Build history of the part. All positions in model axes, mm. A direction names the side the tool comes from. Give positions to 0.01 mm unless a question says otherwise; leave off trailing zeros. Write each loop counter-clockwise with the first axis right and the second up, starting at its lowest first coordinate (ties: lowest second). Pieces come first, ordered by that corner, then holes.
Autodesk Inventor part; units mm, degrees
ref_plane "YZ Plane" through (0, 0, 0) normal (1, 0, 0) x (0, 1, 0)
ref_plane "XZ Plane" through (0, 0, 0) normal (0, 1, 0) x (-1, 0, 0)
ref_plane "XY Plane" through (0, 0, 0) normal (0, 0, 1) x (1, 0, 0)
sketch "Sketch1" plane through (0, 0, 0) normal (0, 1, 0) x (-1, 0, 0)
  line L0 (0, 0) -> (-100, 0)
  line L1 (-100, 0) -> (-100, -100)
  line L2 (-100, -100) -> (0, -100)
  line L3 (0, -100) -> (0, 0)
  dimension "d0" = 100
  dimension "d1" = 100
extrude "base" add sketch "Sketch1" along normal blind 9
sketch "Sketch2" plane through (0, 9, 0) normal (0, 1, 0) x (1, 0, 0)
  circle A0 centre (96, 25) radius 1.75
  line L0 (100, 0) -> (100, 100)
  circle A1 centre (69, 25) radius 1.75
  line L1 (0, 0) -> (100, 0)
  line L2 (100, 50) -> (95, 50)
  circle A2 centre (96, 75) radius 1.75
  circle A3 centre (69, 75) radius 1.75
  line L3 (63, 0) -> (63, 100)
  line L4 (100, 100) -> (0, 100)
  line L5 (100, 25) -> (100, 11)
  line L6 (100, 11) -> (63, 11)
  line L7 (100, 89) -> (63, 89)
  circle A4 centre (82, 25) radius 17.5
  point P0 (63, 89)
  dimension "d6" = 4
  dimension "d7" = 3.5
  dimension "d9" = 3.5
  dimension "d10" = 27
  dimension "d11" = 25
  dimension "d13" = 37
  dimension "d14" = 14
  dimension "d17" = 35
extrude "wheel space" cut sketch "Sketch2" against normal through all contours A0 | L1 L3 L6 A4 L0 | A4 L6 | L3 L4 L0 L7 | A1 | A2 | A3 picked at (84.4264, 10.3619)
sketch "Sketch3" plane through (0, 0, 0) normal (0, 0, 1) x (1, 0, 0)
  line L0 (63, 9) -> (0, 9)
  line L1 (0, 0) -> (0, 9)
  line L2 (63, 0) -> (0, 0)
  line L3 (5, 9) -> (0, 0)
  dimension "d18" = 5
extrude "ramp" cut sketch "Sketch3" against normal through all
sketch "Sketch4" plane through (0, 9, 0) normal (0, 1, 0) x (1, 0, 0)
  circle A0 centre (69, 75) radius 1.75
  circle A1 centre (96, 25) radius 1.75
  circle A2 centre (96, 75) radius 1.75
  circle A3 centre (69, 25) radius 1.75
  line L0 (5, 100) -> (5, 0)
  line L1 (5, 0) -> (63, 0)
  line L2 (63, 0) -> (63, 11)
  line L3 (63, 11) -> (100, 11)
  line L4 (100, 11) -> (100, 89)
  line L5 (100, 89) -> (63, 89)
  line L6 (63, 89) -> (63, 100)
  line L7 (63, 100) -> (5, 100)
  line L8 (63, 100) -> (63, 89)
  line L9 (61, 95) -> (10, 95)
  line L10 (10, 95) -> (10, 5)
  line L11 (10, 5) -> (63, 5)
  line L12 (63, 11) -> (63, 0)
  line L13 (63, 89) -> (61, 89)
  line L14 (61, 89) -> (61, 95)
  line L15 (63, 5) -> (53, 5)
  line L16 (53, 5) -> (53, 7)
  line L17 (53, 7) -> (63, 7)
  line L18 (63, 7) -> (63, 5)
  point P0 (0, 0)
  point P1 (63, 95)
  dimension "d21" = 5
  dimension "d22" = 5
  dimension "d23" = 5
  dimension "d64" = 2
  dimension "d72" = 10
  dimension "d73" = 2
extrude "walls" add sketch "Sketch4" along normal blind 5 contours L7 L6 L13 L14 L9 L10 L11 L2 L1 L0 | L11 L16 L17 L2
sketch "Sketch5" plane through (0, 9, 0) normal (0, 1, 0) x (1, 0, 0)
  line L0 (22.7322, 84.5) -> (12.7322, 84.5)
  line L1 (12.7322, 84.5) -> (12.7322, 44.5)
  line L2 (12.7322, 44.5) -> (22.7322, 44.5)
  line L3 (22.7322, 44.5) -> (22.7322, 84.5)
  line L4 (14.7322, 44.5) -> (20.7322, 44.5)
  line L5 (20.7322, 44.5) -> (20.7322, 55.5)
  line L6 (20.7322, 55.5) -> (14.7322, 55.5)
  line L7 (14.7322, 55.5) -> (14.7322, 44.5)
  line L8 (14.7322, 44.5) -> (20.7322, 55.5) construction
  line L9 (20.7322, 44.5) -> (14.7322, 55.5) construction
  line L10 (10, 5) -> (10, 95)
  circle A0 centre (17.7322, 64) radius 1.75
  line L11 (100, 84.5) -> (90, 84.5)
  line L12 (90, 84.5) -> (90, 44.5)
  line L13 (90, 44.5) -> (100, 44.5)
  line L14 (100, 44.5) -> (100, 84.5)
  line L15 (92, 44.5) -> (98, 44.5)
  line L16 (98, 44.5) -> (98, 55.5)
  line L17 (98, 55.5) -> (92, 55.5)
  line L18 (92, 55.5) -> (92, 44.5)
  line L19 (92, 44.5) -> (98, 55.5) construction
  line L20 (98, 44.5) -> (92, 55.5) construction
  circle A1 centre (95, 64) radius 1.75
  circle A2 centre (96, 75) radius 1.75
  line L21 (100, 11) -> (100, 89)
  circle A3 centre (95, 36) radius 1.75
  circle A4 centre (17.7322, 36) radius 1.75
  line L22 (100, 57.5) -> (90, 57.5)
  line L23 (90, 57.5) -> (90, 42.5)
  line L24 (90, 42.5) -> (100, 42.5)
  line L25 (100, 42.5) -> (100, 57.5)
  line L26 (100, 57.5) -> (90, 42.5) construction
  line L27 (90, 57.5) -> (100, 42.5) construction
  point P0 (0, 0)
  point P1 (17.7322, 50)
  point P2 (10, 50)
  point P3 (17.7322, 50)
  point P4 (95, 50)
  point P5 (95, 50)
  point P6 (95, 50)
  point P7 (17.7322, 50)
  point P8 (92, 44.5)
  point P9 (98, 44.5)
  point P10 (95, 84.5)
  dimension "d26" = 10
  dimension "d27" = 40
  dimension "d28" = 5.5
  dimension "d29" = 6
  dimension "d30" = 11
  dimension "d31" = 3.5
  dimension "d32" = 14
  dimension "d33" = 10
  dimension "d34" = 40
  dimension "d35" = 5.5
  dimension "d36" = 6
  dimension "d37" = 11
  dimension "d38" = 3.5
  dimension "d39" = 14
  dimension "d60" = 3.5
  dimension "d61" = 14
  dimension "d62" = 3.5
  dimension "d63" = 14
  dimension "d65" = 10
  dimension "d66" = 15
extrude "ir sensor" cut sketch "Sketch5" against normal through all contours L2 L7 L6 L5 | A0 | L13 L18 L17 L16 | A1 | A3 | A4
sketch "Sketch8" plane through (0, 14, 0) normal (0, 1, 0) x (1, 0, 0)
  line L0 (61, 89) -> (63, 89)
  line L1 (63, 89) -> (63, 100)
  line L2 (63, 100) -> (5, 100)
  line L3 (5, 100) -> (5, 0)
  line L4 (5, 0) -> (63, 0)
  line L5 (63, 0) -> (63, 7)
  line L6 (63, 7) -> (53, 7)
  line L7 (53, 7) -> (53, 5)
  line L8 (53, 5) -> (10, 5)
  line L9 (10, 5) -> (10, 95)
  line L10 (10, 95) -> (61, 95)
  line L11 (61, 95) -> (61, 89)
  circle A0 centre (7.5, 85) radius 1.25
  circle A1 centre (7.5, 15) radius 1.25
  circle A2 centre (48, 2.5) radius 1.25
  circle A3 centre (48, 97.5) radius 1.25
  point P0 (0, 0)
  dimension "d82" = 2.5
  dimension "d84" = 2.5
  dimension "d85" = 2.5
  dimension "d87" = 2.5
  dimension "d88" = 15
  dimension "d89" = 15
  dimension "d90" = 15
  dimension "d91" = 2.5
  dimension "d92" = 2.5
  dimension "d93" = 2.5
sketch "Sketch6" plane through (0, 9, 0) normal (0, 1, 0) x (1, 0, 0)
  line L0 (20.7322, 44.5) -> (14.7322, 44.5)
  circle A0 centre (17.7322, 64) radius 1.75
  line L1 (53, 5) -> (10, 5)
  line L2 (10, 95) -> (61, 95)
  circle A1 centre (69, 25) radius 1.75
  circle A2 centre (96, 25) radius 1.75
  circle A3 centre (69, 25) radius 1.75
  circle A4 centre (96, 25) radius 1.75
  line L3 (69, 25) -> (96, 25)
  circle A5 centre (30, 25) radius 1.25
  line L4 (10, 5) -> (10, 95)
  circle A6 centre (30, 59.5) radius 1.25
  circle A7 centre (48, 97.5) radius 1.25
  circle A8 centre (48, 2.5) radius 1.25
  circle A9 centre (7.5, 85) radius 1.25
  circle A10 centre (7.5, 15) radius 1.25
  point P0 (0, 0)
  point P1 (63, 5)
  point P2 (63, 95)
  dimension "d75" = 2.5
  dimension "d76" = 20
  dimension "d77" = 20
  dimension "d79" = 2.5
  dimension "d80" = 34.5
extrude "mount holes" cut sketch "Sketch6" against normal through all both and the other way through all contours A5 | A6 | A7 | A8 | A9 | A10
sketch "Sketch7" plane through (0, 0, 0) normal (0, -1, 0) x (1, 0, 0)
  line L0 (92, -44.5) -> (98, -44.5)
  line L1 (98, -44.5) -> (98, -55.5)
  line L2 (98, -55.5) -> (92, -55.5)
  line L3 (92, -55.5) -> (92, -44.5)
  circle A0 centre (17.7322, -64) radius 1.75
  circle A1 centre (95, -64) radius 1.75
  line L4 (20.7322, -44.5) -> (20.7322, -55.5)
  line L5 (20.7322, -55.5) -> (14.7322, -55.5)
  line L6 (14.7322, -55.5) -> (14.7322, -44.5)
  line L7 (14.7322, -44.5) -> (20.7322, -44.5)
  circle A2 centre (69, -75) radius 1.75
  circle A3 centre (96, -25) radius 1.75
  circle A4 centre (96, -75) radius 1.75
  circle A5 centre (69, -25) radius 1.75
  line L8 (63, -100) -> (63, -89)
  line L9 (63, -89) -> (100, -89)
  line L10 (100, -11) -> (100, -89)
  line L11 (100, -11) -> (63, -11)
  line L12 (63, -11) -> (63, 0)
  line L13 (0, 0) -> (63, 0)
  line L14 (0, -100) -> (0, 0)
  line L15 (63, -100) -> (0, -100)
  circle A6 centre (69, -75) radius 6
  circle A7 centre (69, -25) radius 1.75
  circle A8 centre (69, -25) radius 6
  circle A9 centre (96, -25) radius 1.75
  circle A10 centre (17.7322, -64) radius 6
  circle A11 centre (95, -36) radius 1.75
  arc A12 (89, -36) -> (95, -42) centre (95, -36) ccw
  line L16 (98, -31) -> (98.3166, -31)
  line L17 (100, -11) -> (100, -89)
  line L18 (96, -19) -> (100, -19)
  line L19 (100, -50) -> (98.3161, -50)
  line L20 (95, -42) -> (100, -42)
  circle A13 centre (17.7322, -36) radius 1.75
  circle A14 centre (17.7322, -36) radius 6
  line L21 (92, -19) -> (96, -19)
  line L22 (89, -36) -> (89, -19)
  line L23 (89, -19) -> (92, -19)
  circle A15 centre (96, -75) radius 1.75
  circle A16 centre (96, -75) radius 1.75
  circle A17 centre (95, -64) radius 1.75
  arc A18 (95, -58) -> (89, -64) centre (95, -64) ccw
  line L24 (98, -69) -> (98.3166, -69)
  line L25 (96, -81) -> (100, -81)
  line L26 (95, -58) -> (100, -58)
  line L27 (92, -81) -> (96, -81)
  line L28 (89, -64) -> (89, -81)
  line L29 (89, -81) -> (92, -81)
  circle A19 centre (30, -59.5) radius 1.25
  circle A20 centre (30, -25) radius 1.25
  circle A21 centre (30, -59.5) radius 6
  circle A22 centre (30, -25) radius 6
  circle A23 centre (48, -97.5) radius 1.25
  circle A24 centre (48, -2.5) radius 1.25
  circle A25 centre (7.5, -15) radius 1.25
  circle A26 centre (7.5, -85) radius 1.25
  arc A27 (52, -97.5) -> (44, -97.5) centre (48, -97.5) ccw
  line L30 (44, -97.5) -> (44, -100)
  line L31 (63, -100) -> (5, -100)
  line L32 (52, -97.5) -> (52, -100)
  line L33 (44, -2.5) -> (44, 0)
  line L34 (0, 0) -> (63, 0)
  line L35 (52, -2.5) -> (52, 0)
  circle A28 centre (7.5, -15) radius 4
  circle A29 centre (7.5, -85) radius 4
  arc A30 (44, -2.5) -> (52, -2.5) centre (48, -2.5) ccw
  point P0 (100, -31)
  point P1 (96, -31)
  point P2 (93.1644, -30.2877)
  point P3 (96, -69)
  point P4 (93.1644, -69.7123)
  dimension "d69" = 12
  dimension "d71" = 12
  dimension "d94" = 8
  dimension "d96" = 8
  dimension "d97" = 8
extrude "mount holes flush" cut sketch "Sketch7" against normal blind 4 contours L15 L30 A27 L32 | L25 L27 L29 L28 A18 L26 L10 | L20 A12 L22 L23 L21 L18 L10 | L13 L35 A30 L33 | A6 | A8 | A10 | A14 | A20 | A21 | A22 | A28 | A29
extrude "Extrusion8" add sketch "Sketch5" along normal blind 3 contours L14 L13 L16 L17 L18 L12 L22 | L21 L24 L23 L13
properties part number "jeff"
1. Saw through at B-B on z = -75. Give the cut face in (x, y).
2. 3-axis set-ups, long thin cutter, end or side, ignore diameter. For faces 5 (the face through (95, 6, -55.5)), 6 (the face through (94, 4, -30)), 7 (the face through (8, 14, -47)), 8 (the face through (48.1, 2, -93.5)), 9 (the face through (7, 4, -17)): which of +Z, -Z, +X, -X, +Y, -Y reach the whole face in a straight line?
3. Drill centre lines: line 1 along Z through (x, y) = (69, 6.75); line 2 along Z through (x, y) = (48, 13); line 3 along Z through (x, y) = (56, 12). Where is each one in solid material? Low to high.
4. Mould opens along X. For faces 1 (the face through (90.804, 1.972, -59.711)), 2 (the face through (94, 2, -19)), 3 (the face through (47.84, 9.07, -98.74)), 4 (the face through (5, 11, -51)) say: pulls with the +X half, pulls with the -X half, needs draft (parallel to the pull), parting line crosses it, or undercut.
5. Saw through at C-C on x = 68.5. Give the cut face in (y, z), plus the area to 3 significant figures.
6. Saw through at A-A on y = 10.5. Give the cut face in (x, z).
7. Saw through at D-D on z = -39.5. Give the cut face in (x, y).
8. Drop flat-ended pins along their axis: pin 1 (4.5 mm diameter, centred on x = 82.5, y = 5.5, fed in from +Z); pin 2 (7 mm diameter, centred on x = 30, z = -59.5, fed in from +Y); pin 3 (6 mm diameter, centred on x = 16, z = -38, fed in from -Y). Give the stop position or say it passes through.
Outcome:
1. outline: (0, 0) - (63, 0) - (63, 4) - (67.25, 4) - (67.25, 9) - (10, 9) - (10, 14) - (5, 14) - (5, 9) - close; (70.75, 4) - (75, 4) - (75, 0) - (89, 0) - (89, 4) - (94.25, 4) - (94.25, 9) - (70.75, 9) - close; (97.75, 4) - (100, 4) - (100, 9) - (97.75, 9) - close
2. face 5: +Y, -Y
2. face 6: +X, -Y
2. face 7: +Z, -Z, +X, -X, +Y
2. face 8: -Z, -Y
2. face 9: -Y
3. line 1: z = -89 to -76.75, -73.25 to -26.75, -23.25 to -11
3. line 2: z = -100 to -98.75, -96.25 to -95, -5 to -3.75, -1.25 to 0
3. line 3: z = -100 to -95, -7 to 0
4. face 1: pulls with the +X half
4. face 2: needs draft
4. face 3: undercut
4. face 4: pulls with the -X half
5. outline: (0, -89) - (9, -89) - (9, -76.68) - (4, -76.68) - (4, -80.98) - (0, -80.98) - close; (0, -69.02) - (4, -69.02) - (4, -73.32) - (9, -73.32) - (9, -26.68) - (4, -26.68) - (4, -30.98) - (0, -30.98) - close; (0, -19.02) - (4, -19.02) - (4, -23.32) - (9, -23.32) - (9, -11) - (0, -11) - close
5. area: 573 mm2
6. outline: (5, -100) - (63, -100) - (63, -89) - (61, -89) - (61, -95) - (10, -95) - (10, -5) - (53, -5) - (53, -7) - (63, -7) - (63, 0) - (5, 0) - close; (90, -57.5) - (100, -57.5) - (100, -42.5) - (90, -42.5) - close; hole circle Ø2.5 at (7.5, -85); hole circle Ø2.5 at (7.5, -15); hole circle Ø2.5 at (48, -97.5); hole circle Ø2.5 at (48, -2.5); hole (92, -55.5) - (98, -55.5) - (98, -44.5) - (92, -44.5) - close
7. outline: (0, 0) - (12.86, 0) - (12.86, 4) - (22.61, 4) - (22.61, 0) - (90.13, 0) - (90.13, 4) - (100, 4) - (100, 9) - (10, 9) - (10, 14) - (5, 14) - (5, 9) - close
8. pin 1: stops at z = -11
8. pin 2: stops at y = 9
8. pin 3: stops at y = 4
